from build123d import *

# Parameters (mm, degrees)
F1_R      = 5.08
F2_DEPTH  = 63.5
F0_R      = 4.445
F3_DEPTH  = 63.5
F5_DEPTH  = 63.5
F7_DEPTH  = 63.5
F8_DEPTH  = 63.5
F9_DEPTH  = 63.5
F10_DEPTH = 63.5
F12_DEPTH = 63.5


with BuildPart() as f2:
    # F1 (on Right) → F2 (new body)
    with BuildSketch(Plane.YZ):
        Circle(F1_R)
    extrude(amount=F2_DEPTH)

    # F0 (on Right) → F3 (cut)
    with BuildSketch(Plane.YZ):
        Circle(F0_R)
    extrude(amount=F3_DEPTH, mode=Mode.SUBTRACT)

    # F4 (on face) → F5 (join)
    with BuildSketch(Plane(origin=(0, 0, 0), x_dir=(0, -1, 0), z_dir=(-1, 0, 0))):
        with BuildLine():
            Line((1.8586593957, 61.8123754669), (0, 62.23))
            ThreePointArc((0, 62.23), (-5.5607094104, 33.655), (0, 5.08))
            Line((0, 5.08), (2.0170907281, 4.6623754669))
            ThreePointArc((2.0170907281, 4.6623754669), (-3.6228573978, 33.2219599945), (1.8586593957, 61.8123754669))
        make_face()
        with BuildLine():
            ThreePointArc((-5.08, 0), (-33.8404680393, -4.6115411802), (-62.23, 1.905))
            Line((-62.23, 1.905), (-63.1423318884, 0))
            ThreePointArc((-63.1423318884, 0), (-34.1176295925, -6.7962114283), (-4.7137119488, -1.8940220863))
            Line((-4.7137119488, -1.8940220863), (-5.08, 0))
        make_face()
    extrude(amount=-F5_DEPTH)

    # F6 (on face) → F7 (join)
    with BuildSketch(Plane(origin=(0, 0, 0), x_dir=(0, -1, 0), z_dir=(-1, 0, 0))):
        with BuildLine():
            Line((0, -62.23), (3.5446478981, -61.8728125))
            ThreePointArc((3.5446478981, -61.8728125), (10.2934213489, -33.0756984809), (1.8712140684, -4.7228125))
            Line((1.8712140684, -4.7228125), (0, -5.08))
            ThreePointArc((0, -5.08), (7.2193443837, -33.655), (0, -62.23))
        make_face()
    extrude(amount=-F7_DEPTH)

    # F4 (on face) → F8 (join)
    with BuildSketch(Plane(origin=(0, 0, 0), x_dir=(0, -1, 0), z_dir=(-1, 0, 0))):
        with BuildLine():
            Line((1.8586593957, 61.8123754669), (0, 62.23))
            ThreePointArc((0, 62.23), (-5.5607094104, 33.655), (0, 5.08))
            Line((0, 5.08), (2.0170907281, 4.6623754669))
            ThreePointArc((2.0170907281, 4.6623754669), (-3.6228573978, 33.2219599945), (1.8586593957, 61.8123754669))
        make_face()
        with BuildLine():
            ThreePointArc((-5.08, 0), (-33.8404680393, -4.6115411802), (-62.23, 1.905))
            Line((-62.23, 1.905), (-63.1423318884, 0))
            ThreePointArc((-63.1423318884, 0), (-34.1176295925, -6.7962114283), (-4.7137119488, -1.8940220863))
            Line((-4.7137119488, -1.8940220863), (-5.08, 0))
        make_face()
    extrude(amount=-F8_DEPTH)

    # F4 (on face) → F9 (join)
    with BuildSketch(Plane(origin=(0, 0, 0), x_dir=(0, -1, 0), z_dir=(-1, 0, 0))):
        with BuildLine():
            Line((1.8586593957, 61.8123754669), (0, 62.23))
            ThreePointArc((0, 62.23), (-5.5607094104, 33.655), (0, 5.08))
            Line((0, 5.08), (2.0170907281, 4.6623754669))
            ThreePointArc((2.0170907281, 4.6623754669), (-3.6228573978, 33.2219599945), (1.8586593957, 61.8123754669))
        make_face()
        with BuildLine():
            ThreePointArc((-5.08, 0), (-33.8404680393, -4.6115411802), (-62.23, 1.905))
            Line((-62.23, 1.905), (-63.1423318884, 0))
            ThreePointArc((-63.1423318884, 0), (-34.1176295925, -6.7962114283), (-4.7137119488, -1.8940220863))
            Line((-4.7137119488, -1.8940220863), (-5.08, 0))
        make_face()
    extrude(amount=-F9_DEPTH)

    # F4 (on face) → F10 (join)
    with BuildSketch(Plane(origin=(0, 0, 0), x_dir=(0, -1, 0), z_dir=(-1, 0, 0))):
        with BuildLine():
            Line((1.8586593957, 61.8123754669), (0, 62.23))
            ThreePointArc((0, 62.23), (-5.5607094104, 33.655), (0, 5.08))
            Line((0, 5.08), (2.0170907281, 4.6623754669))
            ThreePointArc((2.0170907281, 4.6623754669), (-3.6228573978, 33.2219599945), (1.8586593957, 61.8123754669))
        make_face()
        with BuildLine():
            ThreePointArc((-5.08, 0), (-33.8404680393, -4.6115411802), (-62.23, 1.905))
            Line((-62.23, 1.905), (-63.1423318884, 0))
            ThreePointArc((-63.1423318884, 0), (-34.1176295925, -6.7962114283), (-4.7137119488, -1.8940220863))
            Line((-4.7137119488, -1.8940220863), (-5.08, 0))
        make_face()
    extrude(amount=-F10_DEPTH)

    # F11 (on face) → F12 (join)
    with BuildSketch(Plane(origin=(0, 0, 0), x_dir=(0, -1, 0), z_dir=(-1, 0, 0))):
        with BuildLine():
            Line((62.1130176587, -1.905), (62.1130176587, 0))
            ThreePointArc((62.1130176587, 0), (33.6397368663, 5.978196278), (4.9630176587, 1.0677660203))
            Line((4.9630176587, 1.0677660203), (4.9630176587, -0.8372339797))
            ThreePointArc((4.9630176587, -0.8372339797), (33.6388311261, 4.024718381), (62.1130176587, -1.905))
        make_face()
    extrude(amount=-F12_DEPTH)


solid = f2.part
Here's how the part is built. I have some questions about the finished solid (model axes, mm). A direction names the side the tool comes from. Coordinates: 2 decimals unless noted, no trailing zeros. Order: outer loops, then holes, each group sorted by start corner. A loop starts at its lowest first (then second) coordinate and runs counter-clockwise, first axis right, second up. Notation, with made-up numbers: M 62.25,43 L 79.25,43 A13 cw 79.25,59 Z; hole C 57.25,-23.75 d11. An arc over 180 degrees is marked long. Answer as CSV lines item,"result". Start each with the question number.
1. We'd pull the mould along Y, two halves only. Please class faces 1 (the flat face through (31.306, -1.748, -62.054)), 2 (the flat face through (63.5, -4, -9)), 3 (the cylindrical face through (31.31, 34.54, -6.78)): released by +Y, released by -Y, zero draft, split by the parting line, or undercut.
2. I need wall thicknesses on line 1 (Y direction, x = 33.5, z = -34); line 2 (Y direction, x = 24, z = -9); line 3 (Z direction, x = 54.5, y = -56). Which ranges of each line are inside material? Lowest first, please. Write a range as [from, to].
3. I want a section at C-C, the plane z = 55.5. Write out the boundary of the cut face in (x, y), and give its area (3 significant figures).
4. I want a section at B-B, the plane y = -23.5. Write out the boundary of the cut face in (x, z), and give its area (3 significant figures).
5. For pin 1 (3 mm diameter, centred on x = 28, y = 15, fed in from -Z); pin 2 (2 mm diameter, centred on x = 31.5, z = -40.5, fed in from -Y); pin 3 (10 mm diameter, centred on y = 3.5, z = 43.5, fed in from -X); pin 4 (1.5 mm diameter, centred on x = 47.5, z = 12.5, fed in from -Y), each with a flat end and sliding along its axis, tell me the tip position at first contact or that it passes through.
6. On a 3-axis mill with a long thin cutter (end or side, diameter ignored), from which of +Z, -Z, +X, -X, +Y, -Y can I reach the whole of each face in a straight line? I mean faces 4 (the cylindrical face through (31.31, 2.81, -4.23)), 5 (the cylindrical face through (31.31, -34.05, 5.97)). Say none if no direction works.
7. I want a section at A-A, the plane x = 14. Write out the boundary of the cut face in (y, z) (1 decimal), and give its area (3 significant figures).
Recorded:
1,face 1,"released by -Y"
1,face 2,"zero draft"
1,face 3,"undercut"
2,line 1,"y = [-10.31, -7.22]"
2,line 2,"y = [-4.24, -1.94]"
2,line 3,"z = [0.33, 2.25]"
3,outline,"M 0,0.36 L 63.5,0.36 L 63.5,2.36 L 0,2.36 Z"
3,area,"127 mm2"
4,outline,"M 0,3.56 L 63.5,3.56 L 63.5,5.5 L 0,5.5 Z"
4,area,"124 mm2"
5,pin 1,"stops at z = -5.31"
5,pin 2,"stops at y = -10.12"
5,pin 3,"stops at x = 0"
5,pin 4,"stops at y = 0.47"
6,face 4,"-Z, +X, -X"
6,face 5,"+Z, +X, -X"
7,outline,"M -62.1,-1.9 A78.4 cw -5,-0.8 A5.1 ccw -1.9,-4.7 A57.6 ccw -3.5,-61.9 L 0,-62.2 A60.2 cw 0,-5.1 A5.1 ccw 4.7,-1.9 A75.9 ccw 63.1,0 L 62.2,1.9 A76.2 cw 5.1,0 A5.1 ccw 0,5.1 A76.2 ccw 0,62.2 L -1.9,61.8 A76.2 cw -2,4.7 A5.1 ccw -5,1.1 A77.7 ccw -62.1,0 Z; hole C 0,0 d8.9"
7,area,"536 mm2"
